Input: part model. Units: mm. Frame: model coordinates. Face numbers are marked on the shaded views. Coordinates: 2 decimals unless noted, no trailing zeros. Loops run counter-clockwise (first coordinate to the right, second up) from the corner with the lowest first, then second, coordinate; pieces in that order, holes last. Notation, with made-up numbers: (79.5, -34) - (110.5, -34) arc R24 cw to (110.5, -17) - close; hole circle Ø9 at (-11.75, -15). An arc over 180 degrees is marked (long way). Use one line per item in the form item = value.
from build123d import *

# Parameters (mm, degrees)
SKETCH3_W           = 80
SKETCH3_H           = 50
BOSS_EXTRUDE1_DEPTH = 32
SKETCH4_R           = 2.6
CUT_EXTRUDE1_DEPTH  = 5
SKETCH5_R           = 4
CUT_EXTRUDE2_DEPTH  = 65


with BuildPart() as part:
    # Sketch3 → Boss-Extrude1 (new body)
    with BuildSketch(Plane(origin=(0, 0, 0), x_dir=(1, 0, 0), z_dir=(0, 1, 0))):
        Rectangle(SKETCH3_W, SKETCH3_H)
    extrude(amount=BOSS_EXTRUDE1_DEPTH)

    # Sketch4 → Cut-Extrude1 (cut)
    with BuildSketch(Plane(origin=(0, 32, 0), x_dir=(1, 0, 0), z_dir=(0, 1, 0))):
        with Locations((-30, 15)):
            Circle(SKETCH4_R)
        with Locations((30, 15)):
            Circle(SKETCH4_R)
        with Locations((30, -15)):
            Circle(SKETCH4_R)
        with Locations((-30, -15)):
            Circle(SKETCH4_R)
    extrude(amount=-CUT_EXTRUDE1_DEPTH, mode=Mode.SUBTRACT)

    # Sketch5 → Cut-Extrude2 (cut)
    with BuildSketch(Plane(origin=(0, 0, -25), x_dir=(-1, 0, 0), z_dir=(0, 0, -1))):
        with Locations((-30, 16)):
            Circle(SKETCH5_R)
        with Locations((30, 16)):
            Circle(SKETCH5_R)
    extrude(amount=-CUT_EXTRUDE2_DEPTH, mode=Mode.SUBTRACT)


solid = part.part
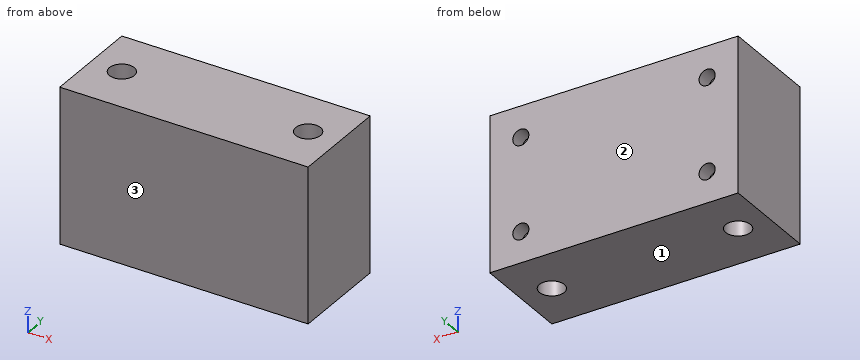
Q1. Pull-direction query (Y, two-part tool) for the marked faces 1, 2 and 3; classes: pulls with the +Y half, pulls with the -Y half, needs draft (parallel to the pull), parting line crosses it, or undercut.
Check values:
face_1 = needs draft
face_2 = pulls with the +Y half
face_3 = pulls with the -Y half
Q2. Ray query, line 1 along Z through (x, y) = (-30, 30.3); line 2 along X through (y, z) = (29.9, -15); line 3 along X through (y, z) = (28, 16). Return the intervals inside material, ascending. Write a range as [from, to].
Check values:
line_1 = [-25, -17.6], [-12.4, 12.4], [17.6, 25]
line_2 = [-40, -32.6], [-27.4, 27.4], [32.6, 40]
line_3 = [-40, -32.4], [-27.6, 27.6], [32.4, 40]
Q3. Cut plane B-B, the plane y = 16. Return loops of the section in (x, z), then the cut area to 3 significant figures.
Check values:
outline = (-40, -25) - (-34, -25) - (-34, 25) - (-40, 25) - close; (-26, -25) - (26, -25) - (26, 25) - (-26, 25) - close; (34, -25) - (40, -25) - (40, 25) - (34, 25) - close
area = 3,200 mm²
Q4. Cut plane D-D, the plane z = 15. Return loops of the section in (x, y).
Check values:
outline = (-40, 0) - (40, 0) - (40, 32) - (32.6, 32) - (32.6, 27) - (27.4, 27) - (27.4, 32) - (-27.4, 32) - (-27.4, 27) - (-32.6, 27) - (-32.6, 32) - (-40, 32) - close; hole circle Ø8 at (-30, 16); hole circle Ø8 at (30, 16)
Q5. First-contact query: P1, Ø6.5, axis at x = 30, y = 16, coming from the -Z side; P2, Ø1.6, axis at x = -30, z = -14.5, coming from the +Y side. Flat tips, straight axial feed; report the tip coordinate or a pass-through.
Check values:
P1 = through
P2 = 27
Q6. Cut plane C-C, the plane x = 30. Return loops of the section in (y, z), then the cut area to 3 significant figures.
Check values:
outline = (0, -25) - (12, -25) - (12, 25) - (0, 25) - close; (20, -25) - (32, -25) - (32, -17.6) - (27, -17.6) - (27, -12.4) - (32, -12.4) - (32, 12.4) - (27, 12.4) - (27, 17.6) - (32, 17.6) - (32, 25) - (20, 25) - close
area = 1,150 mm²
Q7. Cut plane A-A, the plane z = -16. Return loops of the section in (x, y).
Check values:
outline = (-40, 0) - (40, 0) - (40, 32) - (32.4, 32) - (32.4, 27) - (27.6, 27) - (27.6, 32) - (-27.6, 32) - (-27.6, 27) - (-32.4, 27) - (-32.4, 32) - (-40, 32) - close; hole circle Ø8 at (-30, 16); hole circle Ø8 at (30, 16)
